Here's the drawing with two shaded views (mm, measured from the low corner). I have some questions. Round coordinates to 2 decimals unless told otherwise and drop trailing zeros. Loops run counter-clockwise (first coordinate to the right, second up) from the corner with the lowest first, then second, coordinate; pieces in that order, holes last.
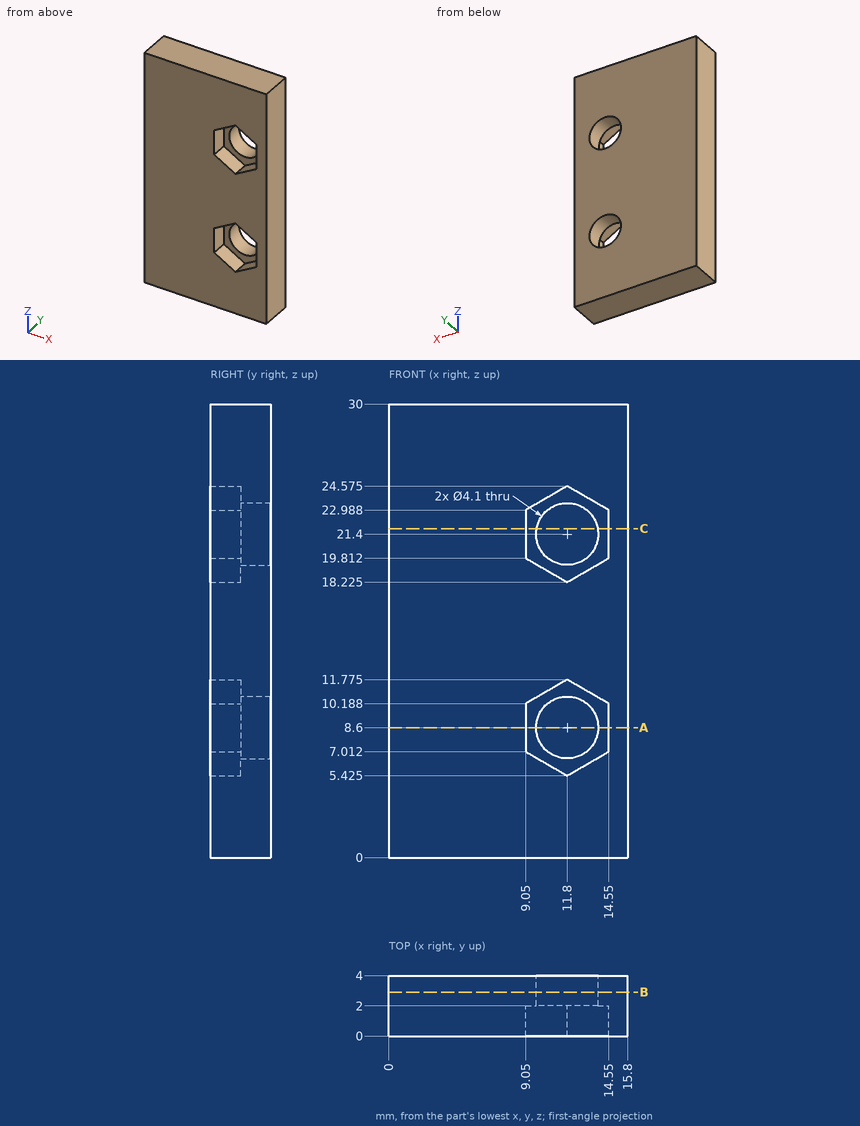
Item 1: If we section it at A-A, the plane z = 8.6: Please give me the cut outline in (x, y), then the cut area to 3 significant figures.
Results list:
outline: (0, 0) - (9.05, 0) - (9.05, 2) - (9.75, 2) - (9.75, 4) - (0, 4) - close; (13.85, 2) - (14.55, 2) - (14.55, 0) - (15.8, 0) - (15.8, 4) - (13.85, 4) - close
area: 44.0 mm2
Item 2: Will these pins go through, and if not, where does the flat tip stop? pin 1 (1.6 mm diameter, centred on x = 13, z = 8.5, fed in from -Y); pin 2 (1 mm diameter, centred on y = 1, z = 20.5, fed in from -X).
Results list:
pin 1: passes through
pin 2: stops at x = 0
Item 3: If we section it at B-B, the plane y = 2.9: Please give me the cut outline in (x, z).
Results list:
outline: (0, 0) - (15.8, 0) - (15.8, 30) - (0, 30) - close; hole circle Ø4.1 at (11.8, 8.6); hole circle Ø4.1 at (11.8, 21.4)
Item 4: If I drill on line 1 along X through (y, z) = (2.8, 8.6); line 2 along Z through (x, y) = (9.25, 1.5) (1 decimal); line 3 along X through (y, z) = (1.3, 10.5), over which ranges is the centre line in solid material (lowest first)?
Results list:
line 1: x = 0 to 9.75, 13.85 to 15.8
line 2: z = 0 to 6.9, 10.3 to 19.7, 23.1 to 30
line 3: x = 0 to 9.59, 14.01 to 15.8
Item 5: If we section it at C-C, the plane z = 21.75: Please give me the cut outline in (x, y).
Results list:
outline: (0, 0) - (9.05, 0) - (9.05, 2) - (9.78, 2) - (9.78, 4) - (0, 4) - close; (13.82, 2) - (14.55, 2) - (14.55, 0) - (15.8, 0) - (15.8, 4) - (13.82, 4) - close
